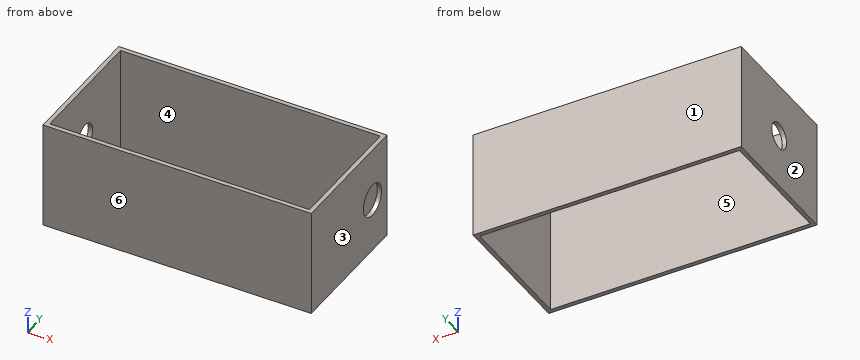
```python
from build123d import *

# Parameters (mm, degrees)
SKIZZE1_W                       = 250
SKIZZE1_H                       = 125
SKIZZE1_W_2                     = 242
SKIZZE1_H_2                     = 117
AUFSATZ_LINEAR_AUSTRAGEN1_DEPTH = 100
SKIZZE2_R                       = 12.25
SCHNITT_LINEAR_AUSTRAGEN1_DEPTH = 10
SKIZZE3_R                       = 15
SCHNITT_LINEAR_AUSTRAGEN2_DEPTH = 10


with BuildPart() as part:
    # Skizze1 → Aufsatz-Linear austragen1 (new body)
    with BuildSketch(Plane.XY):
        with Locations((125, 62.5)):
            Rectangle(SKIZZE1_W, SKIZZE1_H)
        with Locations((125, 62.5)):
            Rectangle(SKIZZE1_W_2, SKIZZE1_H_2, mode=Mode.SUBTRACT)
    extrude(amount=AUFSATZ_LINEAR_AUSTRAGEN1_DEPTH)

    # Skizze2 → Schnitt-Linear austragen1 (cut)
    with BuildSketch(Plane.ZY):
        with Locations((50, 62.5)):
            Circle(SKIZZE2_R)
    extrude(amount=-SCHNITT_LINEAR_AUSTRAGEN1_DEPTH, mode=Mode.SUBTRACT)

    # Skizze3 → Schnitt-Linear austragen2 (cut)
    with BuildSketch(Plane.ZY.offset(-246)):
        with Locations(Location((50, 101, 0), (0, 0, 270))):
            Circle(SKIZZE3_R)
    extrude(amount=-SCHNITT_LINEAR_AUSTRAGEN2_DEPTH, mode=Mode.SUBTRACT)


solid = part.part
```
Read the model definition and answer for the solid it produces. Units are mm, in the model's axes. Face numbers are marked on the shaded views. A direction names the side the tool comes from. Round coordinates to 2 decimals unless told otherwise and drop trailing zeros. Write each loop counter-clockwise with the first axis right and the second up, starting at its lowest first coordinate (ties: lowest second). Pieces come first, ordered by that corner, then holes. Notation, with made-up numbers: (-28, 35.5) -> (11, 35.5) arc R22 cw to (11, 57.5) -> close; hole circle Ø3 at (-39, 47). An arc over 180 degrees is marked (long way). Answer in a Markdown table with one row per item. Add a question column.
1) Given P1, Ø4, axis at y = 82.5, z = 88.5, coming from the -X side, flat-ended and moving along its own axis, determine where the tip first touches the part or whether it passes through.
2) Consider line 1 (Z direction, x = 247, y = 101); line 2 (Y direction, x = 103, z = 91); line 3 (Y direction, x = 0.9, z = 50). Determine where each line is inside the solid, lowest interval first.
3) Which of the six approach directions +Z, -Z, +X, -X, +Y, -Y give full straight-line access (tool end or side, diameter ignored) to the marked faces 5 and 6?
4) Find section A-A, the plane x = 232. Determine the outline of the cut face in (y, z).
5) Find section C-C, the plane z = 50. Determine the outline of the cut face in (x, y).
6) Determine the mould class of the marked faces 1, 2, 3 and 4 for opening direction X: pulls with the +X half, pulls with the -X half, needs draft (parallel to the pull), parting line crosses it, or undercut.
7) Find section D-D, the plane y = 14. Determine the outline of the cut face in (x, z).
8) Find section B-B, the plane y = 101. Determine the outline of the cut face in (x, z), and give its area (3 significant figures).
Findings below:
| question | item | result |
|---|---|---|
| 1 | P1 | x = 0 |
| 2 | line 1 | 0 to 35, 65 to 100 |
| 2 | line 2 | 0 to 4, 121 to 125 |
| 2 | line 3 | 0 to 50.25, 74.75 to 125 |
| 3 | face 5 | +Z, -Z |
| 3 | face 6 | +Z, -Z, +X, -X, -Y |
| 4 | outline | (0, 0) -> (4, 0) -> (4, 100) -> (0, 100) -> close; (121, 0) -> (125, 0) -> (125, 100) -> (121, 100) -> close |
| 5 | outline | (0, 0) -> (250, 0) -> (250, 86) -> (246, 86) -> (246, 4) -> (4, 4) -> (4, 50.25) -> (0, 50.25) -> close; (0, 74.75) -> (4, 74.75) -> (4, 121) -> (246, 121) -> (246, 116) -> (250, 116) -> (250, 125) -> (0, 125) -> close |
| 6 | face 1 | needs draft |
| 6 | face 2 | pulls with the -X half |
| 6 | face 3 | pulls with the +X half |
| 6 | face 4 | undercut |
| 7 | outline | (0, 0) -> (4, 0) -> (4, 100) -> (0, 100) -> close; (246, 0) -> (250, 0) -> (250, 100) -> (246, 100) -> close |
| 8 | outline | (0, 0) -> (4, 0) -> (4, 100) -> (0, 100) -> close; (246, 0) -> (250, 0) -> (250, 35) -> (246, 35) -> close; (246, 65) -> (250, 65) -> (250, 100) -> (246, 100) -> close |
| 8 | area | 680 mm² |
